Autodesk Inventor part; units mm, degrees
ref_plane "YZ Plane" through (0, 0, 0) normal (1, 0, 0) x (0, 1, 0)
ref_plane "XZ Plane" through (0, 0, 0) normal (0, 1, 0) x (-1, 0, 0)
ref_plane "XY Plane" through (0, 0, 0) normal (0, 0, 1) x (1, 0, 0)
sketch "Sketch1" plane through (0, 0, 0) normal (0, 0, 1) x (1, 0, 0)
  circle A0 centre (0, 0) radius 23
  circle A1 centre (0, 0) radius 8
  circle A2 centre (0, 0) radius 2.5
  circle A3 centre (0, 15) radius 3.5
  dimension "d0" = 46
  dimension "d1" = 16
  dimension "d2" = 5
  dimension "d3" = 7
  dimension "d4" = 15
extrude "Extrusion1" add sketch "Sketch1" along normal blind 5 contours A0
extrude "Extrusion2" add sketch "Sketch1" along normal blind 32 contours A1
chamfer "Chamfer1" distance 0.5 angle 45 1 edges at (-8, 0, 32)
chamfer "Chamfer2" distance 0.25 angle 45 2 edges at (-23, 0, 5) (-23, 0, 0)
chamfer "Chamfer3" distance 2 angle 45 1 edges at (-3.5, 15, 0)
properties part number "CylinderCover"
The listing builds one solid part. Answer for the finished solid, in the listing's coordinates (mm). Coordinates: 2 decimals unless noted, no trailing zeros. Loops run counter-clockwise (first coordinate to the right, second up) from the corner with the lowest first, then second, coordinate; pieces in that order, holes last. Notation, with made-up numbers: (77, 88.25) -> (106, 88.25) arc R33 cw to (106, 126.25) -> close; hole circle Ø3 at (30.5, -24.75). An arc over 180 degrees is marked (long way). Answer in a Markdown table with one row per item. Add a question column.
1. Flat-ended cylindrical pins translate along their axes: P1, Ø3, axis at x = 0, y = 0, coming from the +Z side; P2, Ø6, axis at y = 13, z = 3.5, coming from the +X side; P3, Ø8, axis at x = -12.5, y = 17.5, coming from the -Z side; P4, Ø10, axis at x = -12.5, y = 4, coming from the +Z side. Find the tip coordinate at first contact, or state that the pin passes through.
2. The part is cut by section B-B, the plane y = 0. Write down the section's boundary in (x, z), then the cut area to 3 significant figures.
3. The part is cut by section A-A, the plane x = 0. Write down the section's boundary in (y, z).
4. Determine the mould class of faces 1 (the cylindrical face through (-0.54, 2.44, 15.78)), 2 (the flat face through (0, -10, 5)), 3 (the cylindrical face through (-1.73, 7.81, 18.06)) for opening direction X: +X half, -X half, draft (parallel to the pull), parting line (faces both ways), or undercut.
5. Consider line 1 (Y direction, x = 0, z = 2); line 2 (Y direction, x = 0, z = 28.5); line 3 (Z direction, x = 2.5, y = -15). Determine where each line is inside the solid, lowest interval first. Write a range as [from, to].
6. The part is cut by section C-C, the plane z = 23. Write down the section's boundary in (x, y), then the cut area to 3 significant figures.
Answer below:
| question | item | result |
|---|---|---|
| 1 | P1 | through |
| 1 | P2 | x = 20.71 |
| 1 | P3 | z = 0 |
| 1 | P4 | z = 5 |
| 2 | outline | (-23, 0.25) -> (-22.75, 0) -> (-2.5, 0) -> (-2.5, 32) -> (-7.5, 32) -> (-8, 31.5) -> (-8, 5) -> (-22.75, 5) -> (-23, 4.75) -> close; (2.5, 0) -> (22.75, 0) -> (23, 0.25) -> (23, 4.75) -> (22.75, 5) -> (8, 5) -> (8, 31.5) -> (7.5, 32) -> (2.5, 32) -> close |
| 2 | area | 502 mm2 |
| 3 | outline | (-23, 0.25) -> (-22.75, 0) -> (-2.5, 0) -> (-2.5, 32) -> (-7.5, 32) -> (-8, 31.5) -> (-8, 5) -> (-22.75, 5) -> (-23, 4.75) -> close; (2.5, 0) -> (9.5, 0) -> (11.5, 2) -> (11.5, 5) -> (8, 5) -> (8, 31.5) -> (7.5, 32) -> (2.5, 32) -> close; (18.5, 2) -> (20.5, 0) -> (22.75, 0) -> (23, 0.25) -> (23, 4.75) -> (22.75, 5) -> (18.5, 5) -> close |
| 4 | face 1 | undercut |
| 4 | face 2 | draft |
| 4 | face 3 | parting line |
| 5 | line 1 | [-23, -2.5], [2.5, 11.5], [18.5, 23] |
| 5 | line 2 | [-8, -2.5], [2.5, 8] |
| 5 | line 3 | [0, 5] |
| 6 | outline | circle Ø16 at (0, 0); hole circle Ø5 at (0, 0) |
| 6 | area | 181 mm2 |
